Job drawing, mm, ordinate dimensions from the low corner. One solid piece. A direction names the side the tool comes from. Coordinates: 2 decimals unless noted, no trailing zeros. Write each loop counter-clockwise with the first axis right and the second up, starting at its lowest first coordinate (ties: lowest second). Pieces come first, ordered by that corner, then holes.
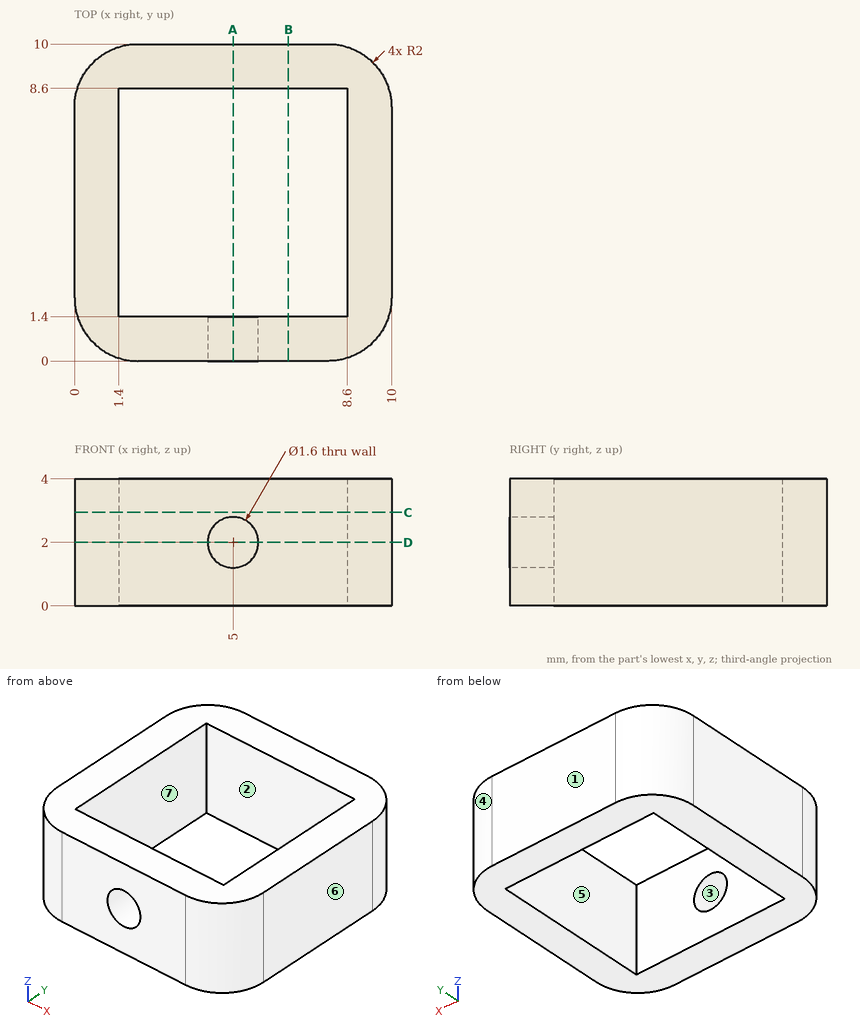
1. Mould opens along Y. For the marked faces 4, 5, 6 and 7 say: +Y half, -Y half, draft (parallel to the pull), parting line (faces both ways), or undercut.
Computed values:
face 4: +Y half
face 5: undercut
face 6: draft
face 7: undercut
2. 3-axis set-ups, long thin cutter, end or side, ignore diameter. For the marked faces 1, 2 and 3: which of +Z, -Z, +X, -X, +Y, -Y reach the whole face in a straight line?
Computed values:
face 1: +Z, -Z, +X, -X, +Y
face 2: +Z, -Z
face 3: -Y
3. Saw through at C-C on z = 2.95. List the corners of the cut face in (x, y).
Computed values:
outline: (0, 2) arc R2 ccw to (2, 0) - (8, 0) arc R2 ccw to (10, 2) - (10, 8) arc R2 ccw to (8, 10) - (2, 10) arc R2 ccw to (0, 8) - close; hole (1.4, 1.4) - (8.6, 1.4) - (8.6, 8.6) - (1.4, 8.6) - close
4. Saw through at D-D on z = 2. List the corners of the cut face in (x, y).
Computed values:
outline: (0, 2) arc R2 ccw to (2, 0) - (4.2, 0) - (4.2, 1.4) - (1.4, 1.4) - (1.4, 8.6) - (8.6, 8.6) - (8.6, 1.4) - (5.8, 1.4) - (5.8, 0) - (8, 0) arc R2 ccw to (10, 2) - (10, 8) arc R2 ccw to (8, 10) - (2, 10) arc R2 ccw to (0, 8) - close
5. Saw through at B-B on x = 6.75. List the corners of the cut face in (y, z).
Computed values:
outline: (0, 0) - (1.4, 0) - (1.4, 4) - (0, 4) - close; (8.6, 0) - (10, 0) - (10, 4) - (8.6, 4) - close
6. Saw through at A-A on x = 5. List the corners of the cut face in (y, z).
Computed values:
outline: (0, 0) - (1.4, 0) - (1.4, 1.2) - (0, 1.2) - close; (0, 2.8) - (1.4, 2.8) - (1.4, 4) - (0, 4) - close; (8.6, 0) - (10, 0) - (10, 4) - (8.6, 4) - close
7. Probe line 1 along Z through (x, y) = (5, 0.95); line 2 along X through (y, z) = (4.25, 1.45). List the from-to ranges inside material, lowest first.
Computed values:
line 1: z = 0 to 1.2, 2.8 to 4
line 2: x = 0 to 1.4, 8.6 to 10
